Check sheet for the drawn part. Datum: minimum x, y, z corner. Units: mm. Round coordinates to 2 decimals unless told otherwise and drop trailing zeros. Loops run counter-clockwise (first coordinate to the right, second up) from the corner with the lowest first, then second, coordinate; pieces in that order, holes last.
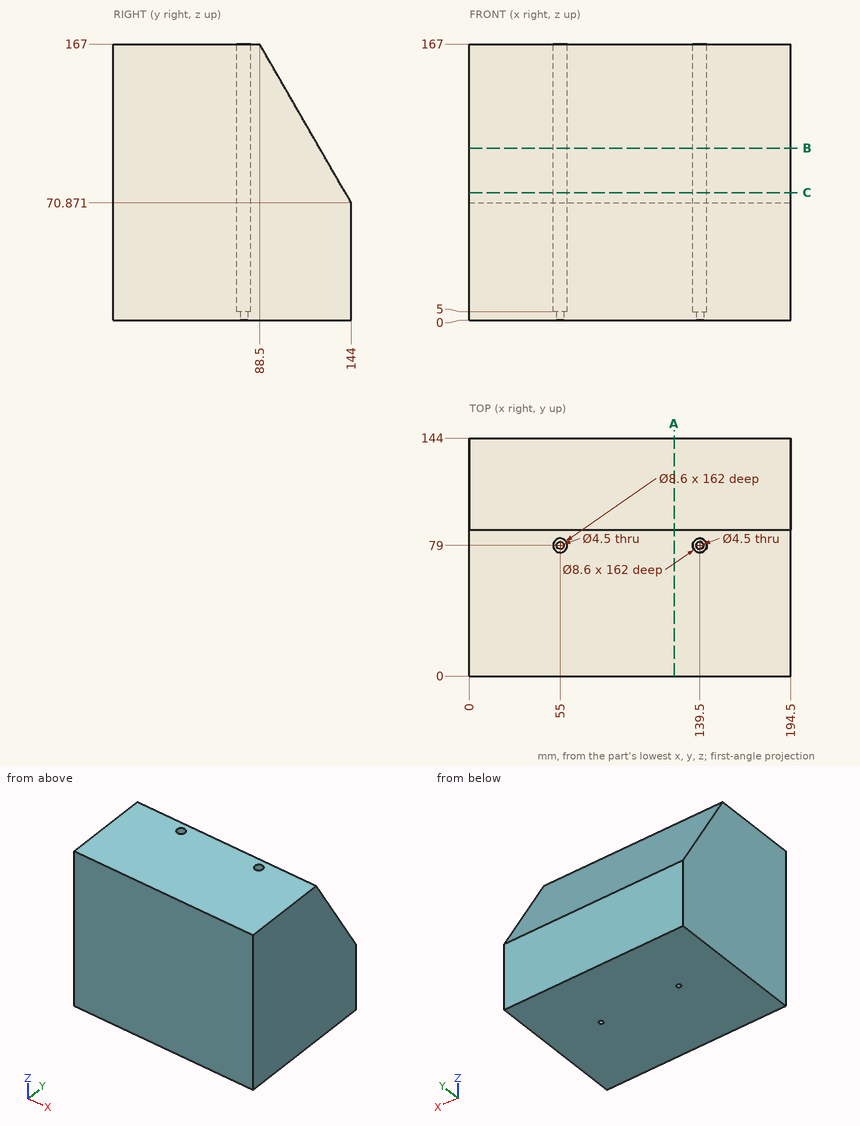
1) Sectioned sample at C-C, the plane z = 77. Record the cut outline in (x, y), then the cut area to 3 significant figures.
Report:
outline: (0, 0) - (194.5, 0) - (194.5, 140.46) - (0, 140.46) - close; hole circle Ø8.6 at (55, 79); hole circle Ø8.6 at (139.5, 79)
area: 27,200 mm2
2) Sectioned sample at A-A, the plane x = 124. Record the cut outline in (y, z), then the cut area to 3 significant figures.
Report:
outline: (0, 0) - (144, 0) - (144, 70.87) - (88.5, 167) - (0, 167) - close
area: 21,400 mm2
3) Gauge pin test, flat end, axial feed: pin 1 (12 mm diameter, centred on x = 34.5, y = 107, fed in from +Z). Record the tip position at first contact, or that the pin passes through.
Report:
pin 1: stops at z = 145.35
4) Scan lines: line 1 along Y through (x, z) = (55, 2.4); line 2 along Y through (x, z) = (55, 65); line 3 along Z through (x, y) = (161.5, 138) (1 decimal). Record each from-to range of solid material in increasing order.
Report:
line 1: y = 0 to 76.75, 81.25 to 144
line 2: y = 0 to 74.7, 83.3 to 144
line 3: z = 0 to 81.3
5) Sectioned sample at B-B, the plane z = 104. Record the cut outline in (x, y).
Report:
outline: (0, 0) - (194.5, 0) - (194.5, 124.87) - (0, 124.87) - close; hole circle Ø8.6 at (55, 79); hole circle Ø8.6 at (139.5, 79)
